Check sheet for the modelled part. Datum: model origin and axes. Units: mm. A direction names the side the tool comes from. Coordinates: 2 decimals unless noted, no trailing zeros. Loops run counter-clockwise (first coordinate to the right, second up) from the corner with the lowest first, then second, coordinate; pieces in that order, holes last. Notation, with made-up numbers: M 54.25,-35.5 L 105.25,-35.5 A18 ccw 105.25,-4.5 Z; hole C 37,32 d5. An arc over 180 degrees is marked long. Write each question's results on one line, items separated by ' | '. Start each with the question number.
from build123d import *

# Parameters (mm, degrees)
SKETCH1_W            = 148.500856602
SKETCH1_H            = 156
BOSS_EXTRUDE1_DEPTH  = 40
FILLET3_R            = 40
FILLET4_R            = 5
SHELL4_T             = -2
SKETCH19_W           = 131
SKETCH19_H           = 146
CUT_EXTRUDE8_DEPTH   = 10
SKETCH21_W           = 107
SKETCH21_H           = 2
BOSS_EXTRUDE7_DEPTH  = 5
BOSS_EXTRUDE8_START  = -107
BOSS_EXTRUDE8_DEPTH  = 107
CUT_EXTRUDE9_DEPTH   = 107
BOSS_EXTRUDE9_DEPTH  = 2
BOSS_EXTRUDE10_DEPTH = 15
CUT_EXTRUDE10_DEPTH  = 170
SHELL5_START         = -57.680419874
SHELL5_DEPTH         = 103
SKETCH29_W           = 7.658063704
SKETCH29_H           = 119.773909492
CUT_EXTRUDE11_DEPTH  = 170
SKETCH31_W           = 7.658063704
SKETCH31_H           = 119.773909492
BOSS_EXTRUDE12_DEPTH = 2
SKETCH32_W           = 7.658063704
SKETCH32_H           = 119.773909492
BOSS_EXTRUDE13_DEPTH = 2
CUT_EXTRUDE12_DEPTH  = 154


# Read off the part's stored shape, not the designer's step: Shell5
# Some blends are built 0.0001 mm under size
with BuildPart() as part:
    # Sketch1 → Boss-Extrude1 (new body)
    with BuildSketch(Plane.XY):
        with Locations((-26.930848175, -80)):
            Rectangle(SKETCH1_W, SKETCH1_H)
    extrude(amount=BOSS_EXTRUDE1_DEPTH)

    # Fillet3
    fillet3_edges = [part.edges().sort_by_distance(p)[0] for p in [
        (-101.181276476, -80, 40),
    ]]
    fillet(fillet3_edges, radius=FILLET3_R - 0.0001)  # a hair under: the kernel refuses the full size

    # Fillet4
    # the kernel refuses this fillet: 5 mm, written as the material it takes off along each edge
    with BuildSketch(Plane(origin=(-61.181376476, -158, 40), x_dir=(0, 1, 0), z_dir=(1, 0, 0))) as fillet4_piece_1:
        with BuildLine():
            CenterArc((FILLET4_R, -FILLET4_R), FILLET4_R, 90, 90)
            Line((0, -FILLET4_R), (0, 0))
            Line((0, 0), (FILLET4_R, 0))
        make_face()
    extrude(amount=121.000956602, mode=Mode.SUBTRACT)
    with BuildSketch(Plane(origin=(-61.181376476, -158, 0.0001), x_dir=(-1, 0, 0), z_dir=(0, 0, -1))) as fillet4_piece_2:
        with BuildLine():
            CenterArc((39.9999 - FILLET4_R, FILLET4_R), FILLET4_R, 270, 90)
            Line((39.9999 - FILLET4_R, 0), (39.9999, 0))
            Line((39.9999, 0), (39.9999, FILLET4_R))
        make_face()
    revolve(axis=Axis((-61.181376476, -158, 0.0001), (0, 1, 0)), revolution_arc=90, mode=Mode.SUBTRACT)
    with BuildSketch(Plane(origin=(-61.181376476, -2, 0.0001), x_dir=(-1, 0, 0), z_dir=(0, 0, -1))) as fillet4_piece_3:
        with BuildLine():
            CenterArc((39.9999 - FILLET4_R, -FILLET4_R), FILLET4_R, 0, 90)
            Line((39.9999, -FILLET4_R), (39.9999, 0))
            Line((39.9999, 0), (39.9999 - FILLET4_R, 0))
        make_face()
    revolve(axis=Axis((-61.181376476, -2, 0.0001), (0, 1, 0)), revolution_arc=90, mode=Mode.SUBTRACT)
    with BuildSketch(Plane(origin=(59.819580126, -2, 40), x_dir=(0, 0, -1), z_dir=(-1, 0, 0))) as fillet4_piece_4:
        with BuildLine():
            CenterArc((FILLET4_R, FILLET4_R), FILLET4_R, 180, 90)
            Line((0, FILLET4_R), (0, 0))
            Line((0, 0), (FILLET4_R, 0))
        make_face()
    extrude(amount=121.000956602, mode=Mode.SUBTRACT)
    with BuildSketch(Plane(origin=(-101.181276476, -2, -12.5), x_dir=(1, 0, 0), z_dir=(0, 0, 1)), Plane(origin=(-101.181276476, -158, -12.5), x_dir=(0, 1, 0), z_dir=(0, 0, 1))) as fillet4_piece_5:
        with BuildLine():
            CenterArc((FILLET4_R, -FILLET4_R), FILLET4_R, 90, 90)
            Line((0, -FILLET4_R), (0, 0))
            Line((0, 0), (FILLET4_R, 0))
        make_face()
    extrude(amount=12.5001, mode=Mode.SUBTRACT)

    # Shell4
    shell4_openings = [part.faces().sort_by_distance(p)[0] for p in [
        (47.319580126, -80, 19.967473228),
    ]]
    offset(amount=SHELL4_T, openings=shell4_openings)

    # Sketch19 → Cut-Extrude8 (cut)
    with BuildSketch(Plane.XY.offset(40)):
        with Locations((-18.180419874, -80)):
            Rectangle(SKETCH19_W, SKETCH19_H)
    extrude(amount=-CUT_EXTRUDE8_DEPTH, mode=Mode.SUBTRACT)

    # Sketch21 → Boss-Extrude7 (add)
    with BuildSketch(Plane(origin=(0, -153, 0), x_dir=(1, 0, 0), z_dir=(0, 1, 0))):
        with Locations((-6.180419874, -39)):
            Rectangle(SKETCH21_W, SKETCH21_H)
    boss_extrude7 = extrude(amount=BOSS_EXTRUDE7_DEPTH)

    # Sketch22 → Boss-Extrude8 (add)
    with BuildSketch(Plane(origin=(47.319580126, 0, 0), x_dir=(0, 0, -1), z_dir=(1, 0, 0)).offset(BOSS_EXTRUDE8_START)):
        with BuildLine():
            Line((-38, -148), (-33, -148))
            Line((-33, -148), (-33, -156))
            Line((-33, -156), (-35, -156))
            ThreePointArc((-35, -156), (-37.121320344, -155.121320344), (-38, -153))
            Line((-38, -153), (-38, -148))
        make_face()
    boss_extrude8 = extrude(amount=BOSS_EXTRUDE8_DEPTH)

    # Sketch23 → Cut-Extrude9 (cut)
    with BuildSketch(Plane(origin=(47.319580126, 0, 0), x_dir=(0, 0, -1), z_dir=(1, 0, 0))):
        Polygon((-37.667948512, -148), (-37.667948512, -152.05), (-33.667948512, -148), align=None)
    cut_extrude9 = extrude(amount=-CUT_EXTRUDE9_DEPTH, mode=Mode.SUBTRACT)

    # Mirror1: Boss-Extrude7, Boss-Extrude8, Cut-Extrude9 across plane
    add(boss_extrude7.mirror(Plane.ZX.offset(-80)))
    add(boss_extrude8.mirror(Plane.ZX.offset(-80)))
    add(cut_extrude9.mirror(Plane.ZX.offset(-80)), mode=Mode.SUBTRACT)

    # Sketch25 → Boss-Extrude9 (add)
    with BuildSketch(Plane(origin=(47.319580126, 0, 0), x_dir=(0, 0, -1), z_dir=(1, 0, 0))):
        Polygon((-40, -148), (-37.667948512, -148), (-37.667948512, -152.05), (-33.667948512, -148), (-33, -148), (-33, -156), (-2, -156), (-2, -4), (-33, -4), (-33, -12), (-33.667948512, -12), (-37.667948512, -7.95), (-37.667948512, -12), (-40, -12), align=None)
    extrude(amount=-BOSS_EXTRUDE9_DEPTH)

    # Sketch26 → Boss-Extrude10 (add)
    with BuildSketch(Plane(origin=(0, 0, 0), x_dir=(-1, 0, 0), z_dir=(0, 0, -1))):
        Polygon((101.181276476, -7), (101.181276476, -153), (101.181276476, -158), (96.181276476, -158), (-47.319580126, -158), (-47.319580126, -2), (96.181276476, -2), (101.181276476, -2), align=None)
    extrude(amount=BOSS_EXTRUDE10_DEPTH)

    # Sketch27 → Cut-Extrude10 (cut)
    with BuildSketch(Plane.ZY.offset(101.181276476)):
        Polygon((-15.241421356, -1.9), (0, -1.9), (0, -2), (0, -17), (0, -17.141421356), align=None)
        Polygon((0, -142.858578644), (-15.241421356, -158.1), (0, -158.1), (0, -158), (0, -143), align=None)
    extrude(amount=-CUT_EXTRUDE10_DEPTH, mode=Mode.SUBTRACT)

    # Shell5 outline → Shell5 (cut)
    with BuildSketch(Plane.YZ.offset(SHELL5_START)):
        with BuildLine():
            Line((-152.194861825, 35), (-154.69858558, 37.472813585))
            ThreePointArc((-154.69858558, 37.472813585), (-155.654784053, 36.397183463), (-156, 35))
            Line((-156, 35), (-152.194861825, 35))
        make_face()
    extrude(amount=SHELL5_DEPTH, mode=Mode.SUBTRACT)

    # Sketch29 → Cut-Extrude11 (cut)
    with BuildSketch(Plane.ZY.offset(101.181276476)):
        with Locations((-8.13310084, -80.031899357)):
            Rectangle(SKETCH29_W, SKETCH29_H)
    extrude(amount=-CUT_EXTRUDE11_DEPTH, mode=Mode.SUBTRACT)

    # Sketch31 → Boss-Extrude12 (add)
    with BuildSketch(Plane(origin=(47.319580126, 0, 0), x_dir=(0, 0, -1), z_dir=(1, 0, 0))):
        with Locations((8.13310084, -80.031899357)):
            Rectangle(SKETCH31_W, SKETCH31_H)
    extrude(amount=-BOSS_EXTRUDE12_DEPTH)

    # Sketch32 → Boss-Extrude13 (add)
    with BuildSketch(Plane.ZY.offset(101.181276476)):
        with Locations((-8.13310084, -80.031899357)):
            Rectangle(SKETCH32_W, SKETCH32_H)
    extrude(amount=-BOSS_EXTRUDE13_DEPTH)

    # Sketch33 → Cut-Extrude12 (cut)
    with BuildSketch(Plane.ZY.offset(101.181276476)):
        Polygon((0, -17.141421356), (0, -17.291421356), (-14.85, -2.441421356), (-14.85, -13.62364303), (-14.85, -146.37635697), (-14.85, -157.558578644), (0, -142.708578644), (0, -142.858578644), (-15, -157.858578644), (-15, -2.141421356), align=None)
    extrude(amount=-CUT_EXTRUDE12_DEPTH, mode=Mode.SUBTRACT)


solid = part.part
1) Thickness scan on probe 1 along Z at (x, y) = (-63, -38.5); probe 2 along Y at (x, z) = (-67, 25.5); probe 3 along X at (y, z) = (-83, -9). Record the ranges inside material, lowest first.
2) Section check B-B (y = -95). Enter the section's corners in (x, z), then the cut area to 3 significant figures.
3) Section check A-A (x = -51). Give the number of separate pieces and of enclosed holes in the cut face, then the cut area to 3 significant figures.
4) Set-up check for faces 1 (the flat face through (-27.97, -9.97, -7.32)), 2 (the flat face through (-28, -81, -4.304)), 3 (the flat face through (-25, -2, 18)): record each of +Z, -Z, +X, -X, +Y, -Y from which the full face is reachable in a straight line by a thin tool's end or side.
5) Gauge pin test, flat ends, axial feed: P1, Ø19, axis at y = -91, z = 22.5, coming from the -X side; P2, Ø3, axis at x = -72.5, z = 36, coming from the +Y side; P3, Ø4, axis at x = -0.5, z = -8.5, coming from the -Y side. Record the tip position at first contact, or that the pin passes through.
6) Release check for a two-part mould opening along Z. For faces 4 (the flat face through (-28, -81, -14.85)), 5 (the flat face through (-28, -81, -11.962)), 6 (the flat face through (46, -80, 40)), 7 (the flat face through (-8, -152, 33)) record: +Z half, -Z half, draft (parallel to the pull), parting line (faces both ways), or undercut.
Return value:
1) probe 1: z = -14.85 to -11.96, -4.3 to 2 | probe 2: y = -158 to -156, -4 to -2 | probe 3: x = -101.18 to -99.18, 45.32 to 47.32
2) outline: M -101.18,-14.85 L 47.32,-14.85 L 47.32,40 L 45.32,40 L 45.32,2 L -99.13,2 A38 cw -83.68,30.62 L -83.68,33.07 A40 ccw -101.18,0 Z; hole M -99.18,-11.96 L 45.32,-11.96 L 45.32,-4.3 L -99.18,-4.3 Z | area: 1,540 mm2
3) separate pieces: 1 | enclosed holes: 2 | area: 1,710 mm2
4) face 1: +X, -X, +Y | face 2: none | face 3: +Z, -Z, +X, -X, +Y
5) P1: stops at x = -99.01 | P2: stops at y = -2.16 | P3: stops at y = -153.21
6) face 4: -Z half | face 5: undercut | face 6: +Z half | face 7: undercut
